from build123d import *

# Parameters (mm, degrees)
ESBO_O1_W                = 12
ESBO_O1_H                = 122
RESSALTO_EXTRUS_O1_DEPTH = 1
ESBO_O2_W                = 12
ESBO_O2_H                = 122
ESBO_O2_W_2              = 10
ESBO_O2_H_2              = 120
RESSALTO_EXTRUS_O2_DEPTH = 10
ESBO_O3_W                = 10
ESBO_O3_H                = 1
RESSALTO_EXTRUS_O3_DEPTH = 11.547005384
PADR_O_START             = -5
PADR_O_LINEAR1_DEPTH     = 10


# Read off the part's stored shape, not the designer's step: Padrão linear1
with BuildPart() as part:
    # Esboço1 → Ressalto-extrusão1 (new body)
    with BuildSketch(Plane.XY):
        Rectangle(ESBO_O1_W, ESBO_O1_H)
    extrude(amount=RESSALTO_EXTRUS_O1_DEPTH)

    # Esboço2 → Ressalto-extrusão2 (add)
    with BuildSketch(Plane.XY.offset(1)):
        Rectangle(ESBO_O2_W, ESBO_O2_H)
        Rectangle(ESBO_O2_W_2, ESBO_O2_H_2, mode=Mode.SUBTRACT)
    extrude(amount=RESSALTO_EXTRUS_O2_DEPTH)

    # Esboço3 → Ressalto-extrusão3 (add, along a direction that is not the sketch's normal)
    with BuildSketch(Plane.XY.offset(1)):
        with Locations((0, 56.5)):
            Rectangle(ESBO_O3_W, ESBO_O3_H)
    extrude(amount=RESSALTO_EXTRUS_O3_DEPTH, dir=(0, -0.4999999999999981, 0.8660254037844398))

    # Padrão linear1 outline → Padrão linear1 (add)
    with BuildSketch(Plane.YZ.offset(PADR_O_START)):
        Polygon((-58.773502692, 11), (-59.773502692, 11), (-54, 1), (-53, 1), align=None)
        Polygon((-48.773502692, 11), (-49.773502692, 11), (-44, 1), (-43, 1), align=None)
        Polygon((-38.773502692, 11), (-39.773502692, 11), (-34, 1), (-33, 1), align=None)
        Polygon((-28.773502692, 11), (-29.773502692, 11), (-24, 1), (-23, 1), align=None)
        Polygon((-18.773502692, 11), (-19.773502692, 11), (-14, 1), (-13, 1), align=None)
        Polygon((-8.773502692, 11), (-9.773502692, 11), (-4, 1), (-3, 1), align=None)
        Polygon((1.226497308, 11), (0.226497308, 11), (6, 1), (7, 1), align=None)
        Polygon((11.226497308, 11), (10.226497308, 11), (16, 1), (17, 1), align=None)
        Polygon((21.226497308, 11), (20.226497308, 11), (26, 1), (27, 1), align=None)
        Polygon((31.226497308, 11), (30.226497308, 11), (36, 1), (37, 1), align=None)
        Polygon((41.226497308, 11), (40.226497308, 11), (46, 1), (47, 1), align=None)
    extrude(amount=PADR_O_LINEAR1_DEPTH)


solid = part.part
Geometry check sheet. Reference: the model listing, model coordinates, mm. A direction names the side the tool comes from. Round coordinates to 2 decimals unless told otherwise and drop trailing zeros. Order: outer loops, then holes, each group sorted by start corner. A loop starts at its lowest first (then second) coordinate and runs counter-clockwise, first axis right, second up. Notation, with made-up numbers: M -7.5,72 L 8.5,72 A17 ccw 8.5,96 Z; hole C 31,-39 d2. An arc over 180 degrees is marked long. Answer in a Markdown table with one row per item. Add a question column.
Item 1: Sectioned sample at C-C, the plane z = 8.5. State how many separate pieces and enclosed holes the cut face has, plus the area to 3 significant figures.
Item 2: Set-up check for faces 4 (the face through (-0.07, -26.927, 6.07)), 5 (the face through (0, 60, 6)), 6 (the face through (0, 1, 0)): record each of +Z, -Z, +X, -X, +Y, -Y from which the full face is reachable in a straight line by a thin tool's end or side.
Item 3: Sectioned sample at A-A, the plane y = -31. Enter the section's corners in (x, z), plus the area to 3 significant figures.
Item 4: Material ranges on L1, parallel to X at y = -8, z = 2.75; L2, parallel to Z at x = -2.25, y = 3.5; L3, parallel to Z at x = 3.25, y = -22, recorded low to high. Write a range as [from, to].
Item 5: Sectioned sample at B-B, the plane y = 15. Enter the section's corners in (x, z).
Item 6: Draft check along Z on faces 1 (the face through (-5, 49, 6)), 2 (the face through (-0.07, -15.846, 5.93)), 3 (the face through (0, -61, 5)). Enter one of: released by +Z, released by -Z, zero draft, split by the parting line, or undercut.
Filled in:
| question | item | result |
|---|---|---|
| 1 | separate pieces | 1 |
| 1 | enclosed holes | 13 |
| 1 | area | 384 mm² |
| 2 | face 4 | none |
| 2 | face 5 | +Z |
| 2 | face 6 | -Z, +X, -X, +Y, -Y |
| 3 | outline | M -6,0 L 6,0 L 6,11 L 5,11 L 5,1 L -5,1 L -5,11 L -6,11 Z |
| 3 | area | 32.0 mm² |
| 4 | L1 | x = [-6, -5], [5, 6] |
| 4 | L2 | z = [0, 1], [5.33, 7.06] |
| 4 | L3 | z = [0, 1] |
| 5 | outline | M -6,0 L 6,0 L 6,11 L 5,11 L 5,4.46 L -5,4.46 L -5,11 L -6,11 Z; hole M -5,1 L 5,1 L 5,2.73 L -5,2.73 Z |
| 6 | face 1 | undercut |
| 6 | face 2 | released by +Z |
| 6 | face 3 | zero draft |
